Geometry: final body of the model. Coordinates: model frame, mm. A direction names the side the tool comes from. Give positions to 0.01 mm unless a question says otherwise; leave off trailing zeros. Write each loop counter-clockwise with the first axis right and the second up, starting at its lowest first coordinate (ties: lowest second). Pieces come first, ordered by that corner, then holes.
from build123d import *

# Parameters (mm, degrees)
SKETCH1_W               = 14
SKETCH1_H               = 14
BOSS_EXTRUDE1_DEPTH     = 7
SKETCH2_W               = 7
SKETCH2_H               = 14
BOSS_EXTRUDE2_DEPTH     = 14
CHAMFER1_SIZE           = 3
CHAMFER2_SIZE           = 0.5
CHAMFER3_SIZE           = 4
CUT_EXTRUDE1_DEPTH      = 28.335873866
CUT_EXTRUDE1_DEPTH_BACK = 28.335873866
SKETCH3_R               = 1.55
SKETCH5_W               = 6.4
SKETCH5_H               = 13
CUT_EXTRUDE2_DEPTH      = 0.54


with BuildPart() as part:
    # Sketch1 → Boss-Extrude1 (new body)
    with BuildSketch(Plane(origin=(0, 0, 0), x_dir=(1, 0, 0), z_dir=(0, 1, 0))):
        with Locations((7, 7)):
            Rectangle(SKETCH1_W, SKETCH1_H)
    extrude(amount=BOSS_EXTRUDE1_DEPTH)

    # Sketch2 → Boss-Extrude2 (add)
    with BuildSketch(Plane(origin=(0, 7, 0), x_dir=(1, 0, 0), z_dir=(0, 1, 0))):
        with Locations((7, 7)):
            Rectangle(SKETCH2_W, SKETCH2_H)
    extrude(amount=BOSS_EXTRUDE2_DEPTH)

    # Chamfer1
    chamfer1_edges = [part.edges().sort_by_distance(p)[0] for p in [
        (3.5, 7, -7),
        (10.5, 7, -7),
    ]]
    chamfer(chamfer1_edges, length=CHAMFER1_SIZE)

    # Chamfer2
    chamfer2_edges = [part.edges().sort_by_distance(p)[0] for p in [
        (0, 7, -7),
        (14, 7, -7),
    ]]
    chamfer(chamfer2_edges, length=CHAMFER2_SIZE - 0.0001)  # a hair under: the kernel refuses the full size

    # Chamfer3
    chamfer3_edges = [part.edges().sort_by_distance(p)[0] for p in [
        (7, 21, 0),
        (7, 21, -14),
    ]]
    chamfer(chamfer3_edges, length=CHAMFER3_SIZE)

    # Sketch3 → Cut-Extrude1 (cut, two sides: drawn at the far end of the back side and taken through both)
    with BuildSketch(Plane(origin=(10.5, 0, 0), x_dir=(0, 0, -1), z_dir=(1, 0, 0)).offset(-CUT_EXTRUDE1_DEPTH_BACK)):
        with Locations((7, 17)):
            Circle(SKETCH3_R)
        with Locations((4, 13)):
            Circle(SKETCH3_R)
        with Locations((4, 3)):
            Circle(SKETCH3_R)
        with Locations((10, 3)):
            Circle(SKETCH3_R)
    extrude(amount=CUT_EXTRUDE1_DEPTH + CUT_EXTRUDE1_DEPTH_BACK, mode=Mode.SUBTRACT)

    # Sketch5 → Cut-Extrude2 (cut)
    with BuildSketch(Plane.XZ):
        with Locations((7, -7)):
            Rectangle(SKETCH5_W, SKETCH5_H)
    extrude(amount=-CUT_EXTRUDE2_DEPTH, mode=Mode.SUBTRACT)


solid = part.part
Q1. Section B-B on y = 13. Output: boundary loops of the cut face in (x, z), plus the area to 3 significant figures.
Filled sheet:
outline: (3.5, -14) - (10.5, -14) - (10.5, -5.55) - (3.5, -5.55) - close; (3.5, -2.45) - (10.5, -2.45) - (10.5, 0) - (3.5, 0) - close
area: 76.3 mm2
Q2. Section D-D on z = -4.75. Count the separate pieces of the cut face and the enclosed holes in it, plus the area to 3 significant figures.
Filled sheet:
separate pieces: 3
enclosed holes: 0
area: 144 mm2
Q3. Ray query, line 1 along Z through (x, y) = (7.5, 4); line 2 along X through (y, z) = (19.5, -9.5); line 3 along Y through (x, z) = (2.75, -9.5). Return the intervals inside material, ascending.
Filled sheet:
line 1: z = -14 to -11.18, -8.82 to -5.18, -2.82 to 0
line 2: x = 3.5 to 10.5
line 3: y = 0 to 1.53, 4.47 to 9.25
Q4. Pin query (flat end, axial travel): P1, Ø1.5, axis at y = 16.5, z = -2, coming from the +X side; P2, Ø4, axis at y = 17, z = -7, coming from the -X side; P3, Ø2, axis at y = 8, z = -5.5, coming from the -X side. Return the tip coordinate at first contact, or that it passes through.
Filled sheet:
P1: stops at x = 10.5
P2: stops at x = 3.5
P3: stops at x = 0.5
Q5. Access query for faces 1 (the flat face through (7, 0.54, -7)), 2 (the flat face through (10.5, 15, -7)), 3 (the flat face through (7, 21, -7)). Directions: +Z, -Z, +X, -X, +Y, -Y. A direction counts if a zero-diameter tool reaches every point of the face in a straight line with its end or side. Return the directions, or none.
Filled sheet:
face 1: -Y
face 2: +Z, -Z, +X, +Y
face 3: +Z, -Z, +X, -X, +Y
Q6. Section C-C on x = 6.5. Output: boundary loops of the cut face in (y, z).
Filled sheet:
outline: (0, -14) - (17, -14) - (21, -10) - (21, -4) - (17, 0) - (0, 0) - (0, -0.5) - (0.54, -0.5) - (0.54, -13.5) - (0, -13.5) - close; hole circle Ø3.1 at (3, -10); hole circle Ø3.1 at (3, -4); hole circle Ø3.1 at (13, -4); hole circle Ø3.1 at (17, -7)
Q7. Pull-direction query (Z, two-part tool) for faces 4 (the flat face through (7, 19, -2)), 5 (the flat face through (3.5, 15, -7)), 6 (the cylindrical face through (6.902, 1.487, -9.664)); classes: released by +Z, released by -Z, zero draft, split by the parting line, or undercut.
Filled sheet:
face 4: released by +Z
face 5: zero draft
face 6: undercut
